Design review of the part built by this model. Coordinates are the model's own, in mm. Face numbers are marked on the shaded views. A direction names the side the tool comes from. Give positions to 0.01 mm unless a question says otherwise; leave off trailing zeros. Write each loop counter-clockwise with the first axis right and the second up, starting at its lowest first coordinate (ties: lowest second). Pieces come first, ordered by that corner, then holes. Notation, with made-up numbers: (10.25, 13) -> (69.25, 13) arc R15 ccw to (69.25, 18) -> close; hole circle Ø6 at (-40, 27). An arc over 180 degrees is marked (long way). Put each result on its own line as item: value. Start each with the question number.
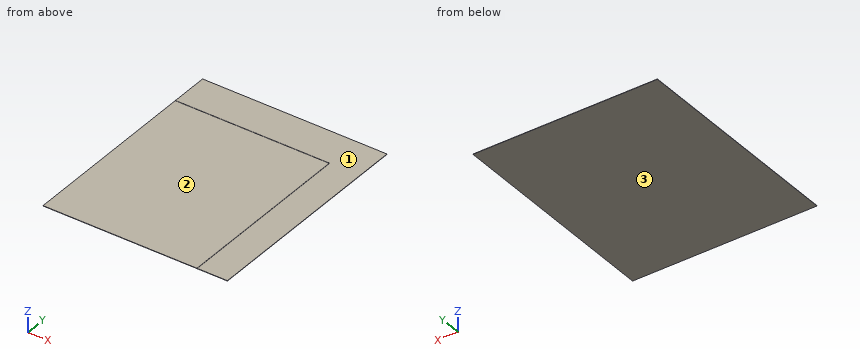
from build123d import *

# Parameters (mm, degrees)
SKETCH1_W           = 1219.2
SKETCH1_H           = 1473.2
BOSS_EXTRUDE1_DEPTH = 2.54
SWEEP1_PROFILE_R    = 1.27


with BuildPart() as part:
    # Sketch1 → Boss-Extrude1 (new body)
    with BuildSketch(Plane.XY):
        Rectangle(SKETCH1_W, SKETCH1_H)
    extrude(amount=BOSS_EXTRUDE1_DEPTH)

    # Sweep1: sweep along a path in Sketch2
    with BuildLine(Plane.XY.offset(2.54)) as sweep1_path:
        Line((408.94, -736.6), (408.94, 482.6))
        ThreePointArc((408.94, 482.6), (408.196051224, 484.396051224), (406.4, 485.14))
        Line((406.4, 485.14), (-609.6, 485.14))
    # Sweep1 profile (on start of the path) → Sweep1 (sweep)
    with BuildSketch(Plane(origin=(408.94, -736.6, 2.54), x_dir=(0, 0, 1), z_dir=(0, 1, 0))):
        Circle(SWEEP1_PROFILE_R)
    sweep(path=sweep1_path.line)


solid = part.part
Q1. Take a section at B-B on x = 153. Give the boundary of the cut face in (y, z), then the cut area to 3 significant figures.
Q2. Take a section at C-C on y = 646. Give the boundary of the cut face in (x, z), then the cut area to 3 significant figures.
Q3. Machinability: for the marked faces 1, 2 and 3, which of the approach directions +Z, -Z, +X, -X, +Y, -Y give a long, thin tool a straight path to every point of the face, cutting with its end or side? Answer none if there is none.
Q4. Take a section at A-A on y = -276.5. Give the boundary of the cut face in (x, z).
Q5. To check wall thickness, follow probe 1 along Z at (x, y) = (458, -379); probe 2 along Y at (x, z) = (-398.5, 2.7); probe 3 along X at (y, z) = (24.5, 2.9). State the ranges of each line that lie inside material, in increasing order. Write a range as from..to.
Result:
1. outline: (-736.6, 0) -> (736.6, 0) -> (736.6, 2.54) -> (486.41, 2.54) arc R1.27 ccw to (483.87, 2.54) -> (-736.6, 2.54) -> close
1. area: 3,740 mm^2
2. outline: (-609.6, 0) -> (609.6, 0) -> (609.6, 2.54) -> (-609.6, 2.54) -> close
2. area: 3,100 mm^2
3. face 1: +Z, +X, +Y
3. face 2: +Z, -X, -Y
3. face 3: -Z, +X, -X, +Y, -Y
4. outline: (-609.6, 0) -> (609.6, 0) -> (609.6, 2.54) -> (410.21, 2.54) arc R1.27 ccw to (407.67, 2.54) -> (-609.6, 2.54) -> close
5. probe 1: z = 0..2.54
5. probe 2: y = 483.88..486.4
5. probe 3: x = 407.72..410.16
